```python
from build123d import *

# Parameters (mm, degrees)
BOSS_EXTRUDE1_DEPTH            = 4.0386
SKETCH2_R                      = 4.7625
BOSS_EXTRUDE2_DEPTH            = 0.508
SKETCH3_R                      = 4.7625
BOSS_EXTRUDE3_DEPTH            = 0.508
CUT_EXTRUDE1_DEPTH             = 1.4986
SKETCH5_W                      = 12.7508
SKETCH5_H                      = 5.715
CUT_EXTRUDE2_DEPTH             = 0.762
SKETCH6_W                      = 3.175
SKETCH6_H                      = 3.2004
CUT_EXTRUDE3_DEPTH             = 1.27
SKETCH7_W                      = 3.175
SKETCH7_H                      = 3.2004
CUT_EXTRUDE4_DEPTH             = 1.27
SKETCH8_W                      = 3.175
SKETCH8_H                      = 2.032
CUT_EXTRUDE5_DEPTH             = 3.1496
SKETCH9_W                      = 3.175
SKETCH9_H                      = 2.032
CUT_EXTRUDE6_DEPTH             = 3.1496
SKETCH10_W                     = 10.16
SKETCH10_H                     = 7.62
CUT_EXTRUDE7_DEPTH             = 5.0386
SKETCH11_W                     = 3.175
SKETCH11_H                     = 2.032
CUT_EXTRUDE8_DEPTH             = 3.556
F_10_CLEARANCE_HOLE1_D         = 5.2324
F_10_CLEARANCE_HOLE1_DEPTH     = 4.5466
F_50_0_07_DIAMETER_HOLE1_D     = 1.778
F_50_0_07_DIAMETER_HOLE1_DEPTH = 3.048
FILLET1_R                      = 0.508
FILLET3_R                      = 2.286
FILLET4_R                      = 3.175
FILLET5_R                      = 9.9187


with BuildPart() as part:
    # Sketch1 → Boss-Extrude1 (new body)
    with BuildSketch(Plane(origin=(0, 2.0193, 0), x_dir=(1, 0, 0), z_dir=(0, 1, 0))):
        with BuildLine():
            Line((-8.93437079, -19.83232), (9.077817244, -19.83232))
            Line((9.077817244, -19.83232), (9.077817244, -8.327843243))
            Line((9.077817244, -8.327843243), (20.330239386, 4.595371256))
            ThreePointArc((20.330239386, 4.595371256), (21.061730892, 12.159996), (14.144827941, 15.308818145))
            Line((14.144827941, 15.308818145), (-5.192523198, 11.533713998))
            Line((-5.192523198, 11.533713998), (-19.708049879, -5.137120292))
            ThreePointArc((-19.708049879, -5.137120292), (-20.347266862, -11.7475), (-14.302901614, -14.499111708))
            Line((-14.302901614, -14.499111708), (-12.995647781, -14.243905122))
            ThreePointArc((-12.995647781, -14.243905122), (-9.183549937, -15.74346998), (-8.93437079, -19.83232))
        make_face()
    extrude(amount=-BOSS_EXTRUDE1_DEPTH)

    # Sketch2 → Boss-Extrude2 (add)
    with BuildSketch(Plane.XZ.offset(2.0193)):
        with Locations((15.397931679, -8.89)):
            Circle(SKETCH2_R)
    extrude(amount=BOSS_EXTRUDE2_DEPTH)

    # Sketch3 → Boss-Extrude3 (add)
    with BuildSketch(Plane.XZ.offset(2.0193)):
        with Locations((-15.397931679, 8.89)):
            Circle(SKETCH3_R)
    extrude(amount=BOSS_EXTRUDE3_DEPTH)

    # Sketch4 → Cut-Extrude1 (cut)
    with BuildSketch(Plane(origin=(0, 2.0193, 0), x_dir=(-1, 0, 0), z_dir=(0, 1, 0))):
        with BuildLine():
            Line((6.3754, 5.363130455), (6.3754, 15.4686))
            Line((6.3754, 15.4686), (-6.3754, 15.4686))
            Line((-6.3754, 15.4686), (-6.3754, 5.363130455))
            ThreePointArc((-6.3754, 5.363130455), (0, -8.3312), (6.3754, 5.363130455))
        make_face()
    extrude(amount=-CUT_EXTRUDE1_DEPTH, mode=Mode.SUBTRACT)

    # Sketch5 → Cut-Extrude2 (cut)
    with BuildSketch(Plane(origin=(0, 0.5207, 0), x_dir=(-1, 0, 0), z_dir=(0, 1, 0))):
        with Locations((0, 12.6111)):
            Rectangle(SKETCH5_W, SKETCH5_H)
    extrude(amount=-CUT_EXTRUDE2_DEPTH, mode=Mode.SUBTRACT)

    # Sketch6 → Cut-Extrude3 (cut)
    with BuildSketch(Plane(origin=(0, -0.2413, 0), x_dir=(-1, 0, 0), z_dir=(0, 1, 0))):
        with Locations((4.2799, 11.3538)):
            Rectangle(SKETCH6_W, SKETCH6_H)
    extrude(amount=-CUT_EXTRUDE3_DEPTH, mode=Mode.SUBTRACT)

    # Sketch7 → Cut-Extrude4 (cut)
    with BuildSketch(Plane(origin=(0, -0.2413, 0), x_dir=(-1, 0, 0), z_dir=(0, 1, 0))):
        with Locations((-4.2799, 11.3538)):
            Rectangle(SKETCH7_W, SKETCH7_H)
    extrude(amount=-CUT_EXTRUDE4_DEPTH, mode=Mode.SUBTRACT)

    # Sketch8 → Cut-Extrude5 (cut)
    with BuildSketch(Plane.XY.offset(9.7536)):
        with Locations((4.2799, -0.4953)):
            Rectangle(SKETCH8_W, SKETCH8_H)
    extrude(amount=-CUT_EXTRUDE5_DEPTH, mode=Mode.SUBTRACT)

    # Sketch9 → Cut-Extrude6 (cut)
    with BuildSketch(Plane.XY.offset(9.7536)):
        with Locations((-4.2799, -0.4953)):
            Rectangle(SKETCH9_W, SKETCH9_H)
    extrude(amount=-CUT_EXTRUDE6_DEPTH, mode=Mode.SUBTRACT)

    # Sketch10 → Cut-Extrude7 (cut, through all)
    with BuildSketch(Plane.XZ.offset(2.0193)):
        Rectangle(SKETCH10_W, SKETCH10_H)
    extrude(amount=-CUT_EXTRUDE7_DEPTH, mode=Mode.SUBTRACT)

    # Sketch11 → Cut-Extrude8 (cut)
    with BuildSketch(Plane.XY.offset(-3.81)):
        with Locations((0, -0.4953)):
            Rectangle(SKETCH11_W, SKETCH11_H)
    extrude(amount=-CUT_EXTRUDE8_DEPTH, mode=Mode.SUBTRACT)

    # #10 Clearance Hole1
    with Locations(Plane(origin=(0, -2.5273, 0), x_dir=(-1, 0, 0), z_dir=(0, -1, 0))):
        with Locations((15.397931679, -8.89), (-15.397931679, 8.89)):
            Hole(F_10_CLEARANCE_HOLE1_D / 2, depth=F_10_CLEARANCE_HOLE1_DEPTH)

    # #50 (0.07) Diameter Hole1
    with Locations(Plane(origin=(0, 0.5207, 0), x_dir=(1, 0, 0), z_dir=(0, 1, 0))):
        with Locations((0, -5.715)):
            Hole(F_50_0_07_DIAMETER_HOLE1_D / 2, depth=F_50_0_07_DIAMETER_HOLE1_DEPTH)

    # Fillet1
    fillet1_edges = [part.edges().sort_by_distance(p)[0] for p in [
        (-5.08, -0.7493, 3.81),
        (5.08, -0.7493, 3.81),
        (5.08, -0.7493, -3.81),
        (-5.08, -0.7493, -3.81),
    ]]
    fillet(fillet1_edges, radius=FILLET1_R)

    # Fillet3
    fillet3_edges = [part.edges().sort_by_distance(p)[0] for p in [
        (9.077817244, 0, 19.83232),
        (-8.93437079, 0, 19.83232),
        (-6.3754, 1.27, 5.363130455),
        (6.3754, 1.27, 5.363130455),
    ]]
    fillet(fillet3_edges, radius=FILLET3_R)

    # Fillet4
    fillet4_edges = [part.edges().sort_by_distance(p)[0] for p in [
        (9.077817244, 0, 8.327843243),
    ]]
    fillet(fillet4_edges, radius=FILLET4_R)

    # Fillet5
    fillet5_edges = [part.edges().sort_by_distance(p)[0] for p in [
        (-5.192523198, 0, -11.533713998),
    ]]
    fillet(fillet5_edges, radius=FILLET5_R)


solid = part.part
```
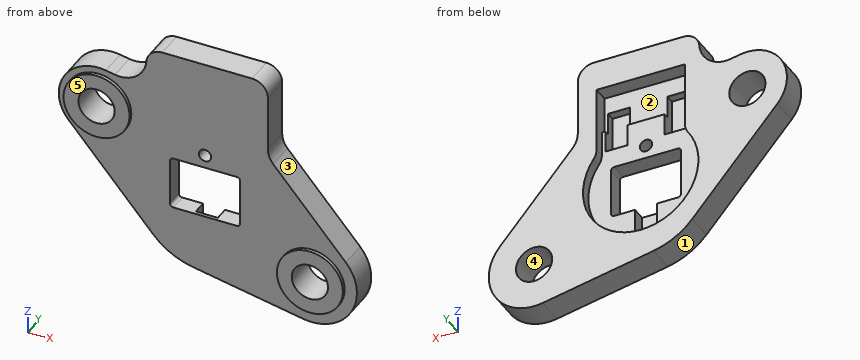
Verification items for the finished model (mm, model axes). Face numbers are marked on the shaded views. A direction names the side the tool comes from. Coordinates: 2 decimals unless noted, no trailing zeros. Write each loop counter-clockwise with the first axis right and the second up, starting at its lowest first coordinate (ties: lowest second). Pieces come first, ordered by that corner, then holes. Notation, with made-up numbers: M 83.5,6 L 106.5,6 A25 ccw 106.5,42 Z; hole C 43,75 d6. An arc over 180 degrees is marked long. One line per item, written item: value.
Item 1: Access from +Z, -Z, +X, -X, +Y, -Y to the whole of each face (thin tool, end or side, straight path). Record for the marked faces 1 and 2.
Check sheet entries:
face 1: -Z, -X, +Y, -Y
face 2: +Y
Item 2: Scan lines: line 1 along Z through (x, y) = (-4, -0.8); line 2 along X through (y, z) = (-0.2, 8.89); line 3 along Z through (x, y) = (0, -0.1). Record each from-to range of solid material in increasing order.
Check sheet entries:
line 1: z = -11.51 to -3.81, 3.81 to 6.6, 12.95 to 19.83
line 2: x = -21.11 to -18.01, -12.78 to -5.87, -2.69 to 2.69, 5.87 to 9.14
line 3: z = -12.55 to -7.37, 3.81 to 4.83, 6.6 to 9.75, 15.47 to 19.83
Item 3: Section check B-B, the plane x = 0. Record the boundary of the cut face in (y, z).
Check sheet entries:
outline: M -2.02,-12.55 L 2.02,-12.55 L 2.02,-8.33 L 0.52,-8.33 L 0.52,-7.37 L -1.51,-7.37 L -1.51,-3.81 L -2.02,-3.81 Z; M -2.02,3.81 L 0.52,3.81 L 0.52,4.83 L -2.02,4.83 Z; M -2.02,6.6 L 0.52,6.6 L 0.52,9.75 L -0.24,9.75 L -0.24,15.47 L 2.02,15.47 L 2.02,19.83 L -2.02,19.83 Z
Item 4: Mould release check, pull along Z, two halves, no side actions. Record for the marked faces 3, 4 and 5: pulls with the +Z half, pulls with the -Z half, needs draft (parallel to the pull), parting line crosses it, or undercut.
Check sheet entries:
face 3: pulls with the +Z half
face 4: undercut
face 5: needs draft
Item 5: Section check D-D, the plane z = 0. Record the boundary of the cut face in (x, y).
Check sheet entries:
outline: M -15.24,-2.02 L -5.08,-2.02 L -5.08,0.52 L -8.33,0.52 L -8.33,2.02 L -15.24,2.02 Z; M 5.08,-2.02 L 16.33,-2.02 L 16.33,2.02 L 8.33,2.02 L 8.33,0.52 L 5.08,0.52 Z
Item 6: Section check A-A, the plane z = 8.89. Record the boundary of the cut face in (x, y).
Check sheet entries:
outline: M -21.11,-2.02 L -20.16,-2.02 L -20.16,-2.53 L -18.01,-2.53 L -18.01,2.02 L -21.11,2.02 Z; M -12.78,-2.53 L -10.64,-2.53 L -10.64,-2.02 L 9.14,-2.02 L 9.14,2.02 L 6.38,2.02 L 6.38,0.52 L 5.87,0.52 L 5.87,-1.51 L 2.69,-1.51 L 2.69,0.52 L -2.69,0.52 L -2.69,-1.51 L -5.87,-1.51 L -5.87,0.52 L -6.38,0.52 L -6.38,2.02 L -12.78,2.02 Z
Item 7: Section check C-C, the plane z = 12.5. Record the boundary of the cut face in (x, y), plus the area to 3 significant figures.
Check sheet entries:
outline: M -19.83,-2.02 L -18.5,-2.02 L -18.5,-2.53 L -12.29,-2.53 L -12.29,-2.02 L 9.08,-2.02 L 9.08,2.02 L 6.38,2.02 L 6.38,-0.24 L 5.87,-0.24 L 5.87,-1.51 L 2.69,-1.51 L 2.69,-0.24 L -2.69,-0.24 L -2.69,-1.51 L -5.87,-1.51 L -5.87,-0.24 L -6.38,-0.24 L -6.38,2.02 L -19.83,2.02 Z
area: 83.0 mm^2
Item 8: Gauge pin test, flat ends, axial feed: pin 1 Ø0.7 at (y, z) = (1, 11.5) entering from +X; pin 2 Ø0.8 at (x, y) = (1, -1) entering from -Z; pin 3 Ø0.6 at (x, y) = (4, -1) entering from -Z. Record the tip position at first contact, or that the pin passes through.
Check sheet entries:
pin 1: stops at x = 9.08
pin 2: stops at z = -12.82
pin 3: stops at z = -13.39
